Part model, mm, in its own coordinate system. Face numbers are marked on the shaded views. A direction names the side the tool comes from. Give positions to 0.01 mm unless a question says otherwise; leave off trailing zeros. Write each loop counter-clockwise with the first axis right and the second up, starting at its lowest first coordinate (ties: lowest second). Pieces come first, ordered by that corner, then holes.
from build123d import *

# Parameters (mm, degrees)
SKETCH_1_W               = 35
SKETCH_1_H               = 80
SKETCH_1_R               = 2.15
EXTRUDE_1_DEPTH          = 30
SKETCH_3_W               = 35
SKETCH_3_H               = 5
EXTRUDE_2_DEPTH          = 40
SKETCH_4_W               = 40
SKETCH_4_H               = 22
SKETCH_4_W_2             = 30
SKETCH_4_H_2             = 20
CUT_EXTRUDE_2_DEPTH      = 70
CHAMFER_1_SIZE           = 5
SKETCH_7_R               = 3.15
CUT_EXTRUDE_3_DEPTH      = 70
CUT_EXTRUDE_4_DEPTH      = 70
SKETCH_9_R               = 2.15
EXTRUDE_3_DEPTH          = 8
EXTRUDE_4_DEPTH          = 35
CUT_EXTRUDE_5_DEPTH      = 154.300358773
CUT_EXTRUDE_5_DEPTH_BACK = 154.300358773
SKETCH_2_R               = 4.1
CUT_EXTRUDE_6_DEPTH      = 179.776396652
CUT_EXTRUDE_6_DEPTH_BACK = 179.776396652
SKETCH_11_W              = 15
SKETCH_11_H              = 156
SKETCH_13_W              = 40
SKETCH_13_H              = 22
CUT_EXTRUDE_7_DEPTH      = 177.453960001
SKETCH_19_W              = 45.998360267
SKETCH_19_H              = 78
CUT_EXTRUDE_11_DEPTH     = 56
SKETCH_21_R              = 2.15
EXTRUDE_8_DEPTH          = 6
SKETCH_22_W              = 39
SKETCH_22_H              = 45
EXTRUDE_9_DEPTH          = 5
SKETCH_23_W              = 20
SKETCH_23_H              = 53
SKETCH_23_R              = 2.15
EXTRUDE_10_DEPTH         = 5


with BuildPart() as part:
    # 草图1 → 凸台-拉伸1 (new body)
    with BuildSketch(Plane(origin=(0, 0, 0), x_dir=(1, 0, 0), z_dir=(0, 1, 0))):
        with Locations((17.5, 40)):
            Rectangle(SKETCH_1_W, SKETCH_1_H)
        with Locations(Location((25, 30, 0), (0, 0, 270))):
            Circle(SKETCH_1_R, mode=Mode.SUBTRACT)
        with Locations(Location((25, 10, 0), (0, 0, 270))):
            Circle(SKETCH_1_R, mode=Mode.SUBTRACT)
    extrude(amount=EXTRUDE_1_DEPTH)

    # 草图3 → 凸台-拉伸2 (add)
    with BuildSketch(Plane(origin=(0, 30, 0), x_dir=(1, 0, 0), z_dir=(0, 1, 0))):
        with Locations((17.5, 42.5)):
            Rectangle(SKETCH_3_W, SKETCH_3_H)
    extrude(amount=EXTRUDE_2_DEPTH)

    # 草图4 → 切除-拉伸2 (cut)
    with BuildSketch(Plane.ZY):
        with Locations((-20, 11)):
            Rectangle(SKETCH_4_W, SKETCH_4_H)
        with Locations((-65, 20)):
            Rectangle(SKETCH_4_W_2, SKETCH_4_H_2)
    extrude(amount=-CUT_EXTRUDE_2_DEPTH, mode=Mode.SUBTRACT)

    # 倒角1
    chamfer_1_edges = [part.edges().sort_by_distance(p)[0] for p in [
        (17.5, 30, -50),
    ]]
    chamfer(chamfer_1_edges, length=CHAMFER_1_SIZE - 0.0001)  # a hair under: the kernel refuses the full size

    # 草图7 → 切除-拉伸3 (cut)
    with BuildSketch(Plane(origin=(0, 0, -45), x_dir=(-1, 0, 0), z_dir=(0, 0, -1))):
        with Locations((-25, 60)):
            Circle(SKETCH_7_R)
        with Locations((-25, 40)):
            Circle(SKETCH_7_R)
    extrude(amount=-CUT_EXTRUDE_3_DEPTH, mode=Mode.SUBTRACT)

    # 草图8 → 切除-拉伸4 (cut)
    with BuildSketch(Plane(origin=(0, 30, 0), x_dir=(1, 0, 0), z_dir=(0, 1, 0))):
        Polygon((0, 0), (15, 0), (0, 36), align=None)
    extrude(amount=-CUT_EXTRUDE_4_DEPTH, mode=Mode.SUBTRACT)

    # 草图9 → 凸台-拉伸3 (add)
    with BuildSketch(Plane(origin=(0, 70, 0), x_dir=(1, 0, 0), z_dir=(0, 1, 0))):
        Polygon((35, 45), (0, 45), (0, 36), (15, 0), (35, 0), align=None)
        with Locations(Location((25, 30, 0), (0, 0, 270))):
            Circle(SKETCH_9_R, mode=Mode.SUBTRACT)
        with Locations(Location((25, 10, 0), (0, 0, 270))):
            Circle(SKETCH_9_R, mode=Mode.SUBTRACT)
    extrude(amount=EXTRUDE_3_DEPTH)

    # 草图10 → 凸台-拉伸4 (add, through all)
    with BuildSketch(Plane.ZY):
        Polygon((-40, 156), (-80, 156), (-80, 146), (-50, 146), (-50, 131), (-45, 126), (-45, 78), (-40.5, 78), align=None)
    extrude(amount=-EXTRUDE_4_DEPTH)

    # 草图2 → 切除-拉伸5 (cut, two sides: drawn at the far end of the back side and taken through both)
    with BuildSketch(Plane(origin=(0, 30, 0), x_dir=(1, 0, 0), z_dir=(0, 1, 0)).offset(-CUT_EXTRUDE_5_DEPTH_BACK)):
        with Locations(Location((10, 70, 0), (0, 0, 270))):
            Circle(SKETCH_2_R)
    extrude(amount=CUT_EXTRUDE_5_DEPTH + CUT_EXTRUDE_5_DEPTH_BACK, mode=Mode.SUBTRACT)

    # 草图11 → 切除-拉伸6 (cut, two sides: drawn at the far end of the back side and taken through both)
    with BuildSketch(Plane.XY.offset(-CUT_EXTRUDE_6_DEPTH_BACK)):
        with Locations((7.5, 78)):
            Rectangle(SKETCH_11_W, SKETCH_11_H)
    extrude(amount=CUT_EXTRUDE_6_DEPTH + CUT_EXTRUDE_6_DEPTH_BACK, mode=Mode.SUBTRACT)

    # 草图13 → 切除-拉伸7 (cut, through all)
    with BuildSketch(Plane(origin=(35, 0, 0), x_dir=(0, 0, -1), z_dir=(1, 0, 0))):
        with Locations((60, 11)):
            Rectangle(SKETCH_13_W, SKETCH_13_H)
    extrude(amount=-CUT_EXTRUDE_7_DEPTH, mode=Mode.SUBTRACT)

    # 草图19 → 切除-拉伸11 (cut)
    with BuildSketch(Plane.ZY.offset(-15)):
        with Locations((-57.000819867, 117)):
            Rectangle(SKETCH_19_W, SKETCH_19_H)
    extrude(amount=-CUT_EXTRUDE_11_DEPTH, mode=Mode.SUBTRACT)

    # 草图21 → 凸台-拉伸8 (add)
    with BuildSketch(Plane(origin=(0, 0, -45), x_dir=(-1, 0, 0), z_dir=(0, 0, -1))):
        Polygon((-35, 78), (-35, 208), (-5, 208), (-5, 158), (-15, 143), (-15, 78), align=None)
        with Locations((-28.5, 201)):
            Circle(SKETCH_21_R, mode=Mode.SUBTRACT)
        with Locations((-14.5, 201)):
            Circle(SKETCH_21_R, mode=Mode.SUBTRACT)
        with Locations((-28.5, 169)):
            Circle(SKETCH_21_R, mode=Mode.SUBTRACT)
        with Locations((-14.5, 169)):
            Circle(SKETCH_21_R, mode=Mode.SUBTRACT)
    extrude(amount=-EXTRUDE_8_DEPTH)

    # 草图22 → 凸台-拉伸9 (add)
    with BuildSketch(Plane(origin=(35, 0, 0), x_dir=(0, 0, -1), z_dir=(1, 0, 0))):
        with Locations((19.5, 100.5)):
            Rectangle(SKETCH_22_W, SKETCH_22_H)
    extrude(amount=-EXTRUDE_9_DEPTH)

    # 草图23 → 凸台-拉伸10 (add)
    with BuildSketch(Plane.XY):
        with Locations((25, 96.5)):
            Rectangle(SKETCH_23_W, SKETCH_23_H)
        with Locations((25, 95)):
            Circle(SKETCH_23_R, mode=Mode.SUBTRACT)
    extrude(amount=-EXTRUDE_10_DEPTH)


solid = part.part
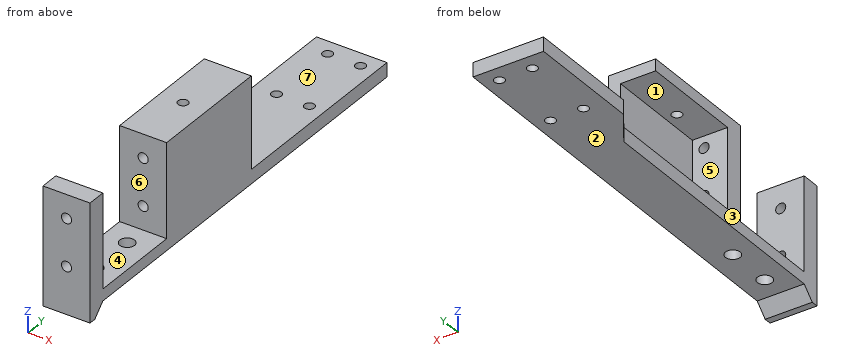
1) 3-axis set-ups, long thin cutter, end or side, ignore diameter. For the marked faces 1, 2, 3 and 4: which of +Z, -Z, +X, -X, +Y, -Y reach the whole face in a straight line?
Check result:
face 1: -X, +Y
face 2: -Z, +X, -X, +Y
face 3: +Z, -Z, -X, -Y
face 4: +Z, +X, -X
2) Mould opens along Y. For the marked faces 5, 6 and 7 say: +Y half, -Y half, draft (parallel to the pull), parting line (faces both ways), or undercut.
Check result:
face 5: +Y half
face 6: undercut
face 7: draft
3) Flat gauge pins, fed straight in: P1, Ø7, axis at x = 25, y = 95, coming from the -Z side; P2, Ø1.5, axis at x = 10, y = 182, coming from the +Z side; P3, Ø16.5, axis at x = 24, z = -24, coming from the +Y side. Where does each tip first touch, or does it go through?
Check result:
P1: stops at z = -45
P2: stops at z = -39
P3: stops at y = 123
4) Drill centre lines: L1, parallel to X at y = 201, z = -43.35; L2, parallel to Y at x = 21, z = -37; L3, parallel to Z at x = 24.25, y = 76. Where is each one in solid material? Low to high.
Check result:
L1: x = 5 to 12.35, 16.65 to 26.35, 30.65 to 35
L2: y = 22 to 30, 70 to 78
L3: z = -45 to -32.01, -27.99 to -12.01, -7.99 to 0
5) Saw through at C-C (y = 95). Write the cut outline in (x, z).
Check result:
outline: (15, -45) - (35, -45) - (35, 0) - (27.15, 0) - (27.15, -5) - (30, -5) - (30, -39) - (15, -39) - close; (15, -5) - (22.85, -5) - (22.85, 0) - (15, 0) - close
6) Saw through at D-D (y = 40). Write the cut outline in (x, z).
Check result:
outline: (15, -45) - (21.85, -45) - (21.85, -40) - (15, -40) - close; (28.15, -45) - (35, -45) - (35, -40) - (28.15, -40) - close
7) Saw through at B-B (y = 169). Write the cut outline in (x, z).
Check result:
outline: (5, -45) - (12.35, -45) - (12.35, -39) - (5, -39) - close; (16.65, -45) - (26.35, -45) - (26.35, -39) - (16.65, -39) - close; (30.65, -45) - (35, -45) - (35, -39) - (30.65, -39) - close
8) Saw through at A-A (z = -30). Write the cut outline in (x, y), and give its area (3 significant figures).
Check result:
outline: (15, 22) - (22.85, 22) - (22.85, 30) - (15, 30) - close; (15, 70) - (22.85, 70) - (22.85, 78) - (15, 78) - close; (27.15, 22) - (35, 22) - (35, 30) - (27.15, 30) - close; (27.15, 70) - (35, 70) - (35, 123) - (30, 123) - (30, 78) - (27.15, 78) - close
area: 476 mm2
